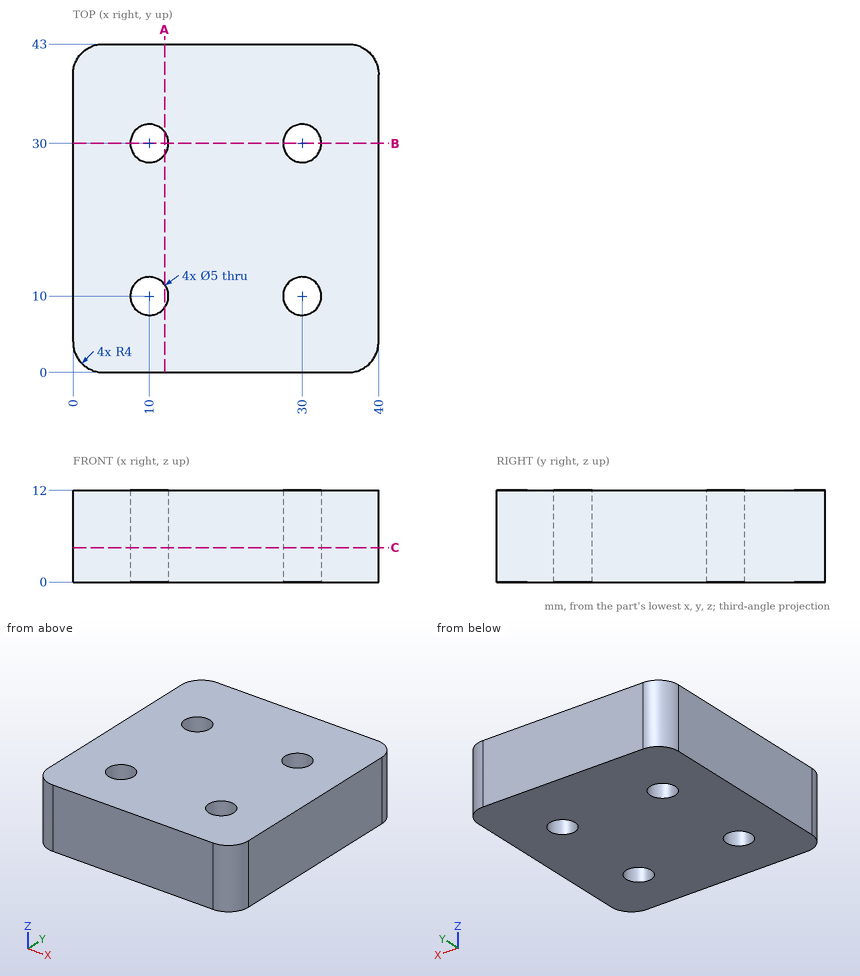
The drawing under review shows one solid part. Ordinate dimensions are in mm from its lowest x, y, z. Coordinates: 2 decimals unless noted, no trailing zeros. Loops run counter-clockwise (first coordinate to the right, second up) from the corner with the lowest first, then second, coordinate; pieces in that order, holes last. Notation, with made-up numbers: (11.25, 32) -> (56.25, 32) arc R18 cw to (56.25, 67) -> close; hole circle Ø5 at (20, 77.5). An arc over 180 degrees is marked (long way). Answer as a JSON object with one key per item and string values.
Q1. Take a section at A-A on x = 12. Give the boundary of the cut face in (y, z).
Answer block:
{"outline": "(0, 0) -> (8.5, 0) -> (8.5, 12) -> (0, 12) -> close; (11.5, 0) -> (28.5, 0) -> (28.5, 12) -> (11.5, 12) -> close; (31.5, 0) -> (43, 0) -> (43, 12) -> (31.5, 12) -> close"}
Q2. To check wall thickness, follow L1, parallel to Y at x = 10, z = 7.5; L2, parallel to Y at x = 29, z = 4.5; L3, parallel to Y at x = 2, z = 4. State the ranges of each line that lie inside material, in increasing order.
Answer block:
{"L1": "y = 0 to 7.5, 12.5 to 27.5, 32.5 to 43", "L2": "y = 0 to 7.71, 12.29 to 27.71, 32.29 to 43", "L3": "y = 0.54 to 42.46"}
Q3. Take a section at C-C on z = 4.5. Give the boundary of the cut face in (x, y).
Answer block:
{"outline": "(0, 4) arc R4 ccw to (4, 0) -> (36, 0) arc R4 ccw to (40, 4) -> (40, 39) arc R4 ccw to (36, 43) -> (4, 43) arc R4 ccw to (0, 39) -> close; hole circle Ø5 at (10, 10); hole circle Ø5 at (10, 30); hole circle Ø5 at (30, 10); hole circle Ø5 at (30, 30)"}
Q4. Take a section at B-B on y = 30. Give the boundary of the cut face in (x, z), plus the area to 3 significant figures.
Answer block:
{"outline": "(0, 0) -> (7.5, 0) -> (7.5, 12) -> (0, 12) -> close; (12.5, 0) -> (27.5, 0) -> (27.5, 12) -> (12.5, 12) -> close; (32.5, 0) -> (40, 0) -> (40, 12) -> (32.5, 12) -> close", "area": "360 mm^2"}
Q5. Clearance check with a flat-ended pin moving along its axis: pin 1 Ø8 at (x, y) = (13.5, 35) entering from -Z. State where the tip first meets the part, or that it passes through.
Answer block:
{"pin 1": "stops at z = 0"}
